from build123d import *

# Parameters (mm, degrees)
SKETCH1_W           = 35.56
SKETCH1_H           = 38.1
BOSS_EXTRUDE1_DEPTH = 6.35
SKETCH2_W           = 6.35
SKETCH2_H           = 12.7
CUT_EXTRUDE1_DEPTH  = 27.820764344
SKETCH3_R           = 2.0955
CUT_EXTRUDE2_DEPTH  = 27.820764344
SKETCH4_R           = 2.0955
CUT_EXTRUDE3_DEPTH  = 27.820764344


with BuildPart() as part:
    # Sketch1 → Boss-Extrude1 (new body)
    with BuildSketch(Plane.XY):
        Rectangle(SKETCH1_W, SKETCH1_H)
    extrude(amount=BOSS_EXTRUDE1_DEPTH)

    # Sketch2 → Cut-Extrude1 (cut, through all)
    with BuildSketch(Plane.XY.offset(6.35)):
        with Locations((14.605, -12.7)):
            Rectangle(SKETCH2_W, SKETCH2_H)
        with Locations((14.605, 12.7)):
            Rectangle(SKETCH2_W, SKETCH2_H)
        with Locations((-14.605, 12.7)):
            Rectangle(SKETCH2_W, SKETCH2_H)
        with Locations((-14.605, -12.7)):
            Rectangle(SKETCH2_W, SKETCH2_H)
    extrude(amount=-CUT_EXTRUDE1_DEPTH, mode=Mode.SUBTRACT)

    # Sketch3 → Cut-Extrude2 (cut, through all)
    with BuildSketch(Plane.XY.offset(6.35)):
        with Locations((14.605, 0)):
            Circle(SKETCH3_R)
        with Locations((-14.605, 0)):
            Circle(SKETCH3_R)
    extrude(amount=-CUT_EXTRUDE2_DEPTH, mode=Mode.SUBTRACT)

    # Sketch4 → Cut-Extrude3 (cut, through all)
    with BuildSketch(Plane.XY.offset(6.35)):
        Circle(SKETCH4_R)
    extrude(amount=-CUT_EXTRUDE3_DEPTH, mode=Mode.SUBTRACT)


solid = part.part
Part model, mm, in its own coordinate system. A direction names the side the tool comes from. Give positions to 0.01 mm unless a question says otherwise; leave off trailing zeros. Order: outer loops, then holes, each group sorted by start corner. A loop starts at its lowest first (then second) coordinate and runs counter-clockwise, first axis right, second up. Notation, with made-up numbers: (35.5, 66) -> (75.5, 66) arc R20 ccw to (75.5, 88) -> close; hole circle Ø2 at (-14.75, -0.5). An arc over 180 degrees is marked (long way). Use one line per item in the form item = value.
(1) Saw through at A-A (x = 0). Write the cut outline in (y, z), then the cut area to 3 significant figures.
Solution:
outline = (-19.05, 0) -> (-2.1, 0) -> (-2.1, 6.35) -> (-19.05, 6.35) -> close; (2.1, 0) -> (19.05, 0) -> (19.05, 6.35) -> (2.1, 6.35) -> close
area = 215 mm²
(2) Drill centre lines: line 1 (Y direction, x = 0, z = 1.5); line 2 (X direction, y = -1, z = 1.5); line 3 (Y direction, x = -14.5, z = 2.5). Where is each one in solid material? Low to high. Write a range as from..to.
Solution:
line_1 = -19.05..-2.1, 2.1..19.05
line_2 = -17.78..-16.45, -12.76..-1.84, 1.84..12.76, 16.45..17.78
line_3 = -6.35..-2.09, 2.09..6.35
(3) Tool access for faces 4 (the face through (11.43, -13, 3)), 5 (the face through (11.43, 13, 3)), 6 (the face through (-15, 6.35, 3)), 7 (the face through (-11.43, -13, 3)): list every direction of +Z, -Z, +X, -X, +Y, -Y with a clear straight run to the whole face (end or side of a thin tool).
Solution:
face_4 = +Z, -Z, +X, -Y
face_5 = +Z, -Z, +X, +Y
face_6 = +Z, -Z, -X, +Y
face_7 = +Z, -Z, -X, -Y
(4) Saw through at C-C (z = 3.5). Count the separate pieces of the cut face and the enclosed holes in it, then the cut area to 3 significant figures.
Solution:
separate_pieces = 1
enclosed_holes = 3
area = 991 mm²
(5) Pull direction Y, two halves, no side cores. Call faces 1 (the face through (17.78, 0, 3)), 2 (the face through (15, -6.35, 3)), 3 (the face through (-16.268, -1.275, 3.219)): +Y half, -Y half, draft (parallel to the pull), parting line (faces both ways), or undercut.
Solution:
face_1 = draft
face_2 = -Y half
face_3 = undercut
(6) Saw through at D-D (x = 15). Write the cut outline in (y, z), then the cut area to 3 significant figures.
Solution:
outline = (-6.35, 0) -> (-2.06, 0) -> (-2.06, 6.35) -> (-6.35, 6.35) -> close; (2.06, 0) -> (6.35, 0) -> (6.35, 6.35) -> (2.06, 6.35) -> close
area = 54.5 mm²
(7) Flat gauge pins, fed straight in: P1, Ø5, axis at x = -14.605, y = 0, coming from the +Z side; P2, Ø1.9, axis at x = 15.5, z = 1.5, coming from the +Y side; P3, Ø3, axis at y = 13, z = 3, coming from the -X side; P4, Ø3, axis at x = -14.5, z = 2.5, coming from the -Y side. Where does each tip first touch, or does it go through?
Solution:
P1 = 6.35
P2 = 6.35
P3 = -11.43
P4 = -6.35
(8) Saw through at B-B (y = 0). Write the cut outline in (x, z).
Solution:
outline = (-17.78, 0) -> (-16.7, 0) -> (-16.7, 6.35) -> (-17.78, 6.35) -> close; (-12.51, 0) -> (-2.1, 0) -> (-2.1, 6.35) -> (-12.51, 6.35) -> close; (2.1, 0) -> (12.51, 0) -> (12.51, 6.35) -> (2.1, 6.35) -> close; (16.7, 0) -> (17.78, 0) -> (17.78, 6.35) -> (16.7, 6.35) -> close
